```python
from build123d import *

# Parameters (mm, degrees)
F0_R     = 57
F0_R_2   = 55
F1_DEPTH = 65
F3_R     = 2.1
F4_DEPTH = 70
F5_R     = 2.1
F6_DEPTH = 100


with BuildPart() as f1:
    # F0 (on Front) → F1 (new body, symmetric)
    with BuildSketch(Plane.XZ):
        with Locations((11.197514832, 9.3730366789)):
            Circle(F0_R)
        with Locations((11.197514832, 9.3730366789)):
            Circle(F0_R_2, mode=Mode.SUBTRACT)
    extrude(amount=F1_DEPTH, both=True)

    # F3 (on plane+point) → F4 (cut, symmetric)
    with BuildSketch(Plane.YZ.offset(11.197514832)):
        with Locations((0, 9.3730366789)):
            Circle(F3_R)
    extrude(amount=F4_DEPTH, both=True, mode=Mode.SUBTRACT)

    # F5 (on Top) → F6 (cut, symmetric)
    with BuildSketch(Plane.XY):
        with Locations((11.197514832, 0)):
            Circle(F5_R)
    extrude(amount=F6_DEPTH, both=True, mode=Mode.SUBTRACT)


solid = f1.part
```
For this review, take the finished solid that the model builds, in its own axes (mm). Round coordinates to 2 decimals unless told otherwise and drop trailing zeros. Order: outer loops, then holes, each group sorted by start corner. A loop starts at its lowest first (then second) coordinate and runs counter-clockwise, first axis right, second up.
Q1. We need section D-D, the plane y = -22. Give the boundary of the cut face in (x, z).
Findings below:
outline: circle Ø114 at (11.2, 9.37); hole circle Ø110 at (11.2, 9.37)
Q2. Mouldability with a two-part tool opening along X and no side actions: class faces 1 (the cylindrical face through (-1.16, -0.91, -46.27)), 2 (the cylindrical face through (67.192, 1.129, 11.144)), 3 (the cylindrical face through (36.58, 0.91, -39.42)) as pulls with the +X half, pulls with the -X half, needs draft (parallel to the pull), parting line crosses it, or undercut.
Findings below:
face 1: parting line crosses it
face 2: needs draft
face 3: undercut
Q3. We need section B-B, the plane x = 40. Give the boundary of the cut face in (y, z), plus the area to 3 significant figures.
Findings below:
outline: (-65, -39.81) - (65, -39.81) - (65, -37.48) - (-65, -37.48) - close; (-65, 56.23) - (65, 56.23) - (65, 58.56) - (-65, 58.56) - close
area: 606 mm2
Q4. Insertion check: P1, Ø6, axis at y = -9.5, z = 28.5, coming from the +X side; P2, Ø1.5, axis at y = 30, z = 8, coming from the -X side; P3, Ø8, axis at x = -33.5, y = -30.5, coming from the -Z side; P4, Ø3.5, axis at y = 0, z = 9.37, coming from the +X side. Each pin has a flat end and moves straight along its axis. Give the tip position at first contact, or say it passes through.
Findings below:
P1: stops at x = 65.87
P2: stops at x = -45.8
P3: stops at z = -30.54
P4: passes through
Q5. Wall thickness on line 1 (X direction, y = -16.5, z = 8.5); line 2 (X direction, y = -5.5, z = 6.5); line 3 (Z direction, x = 43.5, y = 47.5): over which ranges is each line inside the solid? List them lowest first.
Findings below:
line 1: x = -45.8 to -43.8, 66.19 to 68.19
line 2: x = -45.73 to -43.73, 66.12 to 68.13
line 3: z = -37.59 to -35.14, 53.89 to 56.34
Q6. We need section A-A, the plane z = 28.5. Give the boundary of the cut face in (x, y), plus the area to 3 significant figures.
Findings below:
outline: (-42.5, -65) - (-40.37, -65) - (-40.37, 65) - (-42.5, 65) - close; (62.76, -65) - (64.89, -65) - (64.89, 65) - (62.76, 65) - close
area: 553 mm2
Q7. We need section C-C, the plane y = 0. Give the boundary of the cut face in (x, z).
Findings below:
outline: (-45.76, 7.27) arc R57 ccw to (9.1, -47.59) - (9.1, -45.59) arc R55 cw to (-43.76, 7.27) - close; (-45.76, 11.47) - (-43.76, 11.47) arc R55 cw to (9.1, 64.33) - (9.1, 66.33) arc R57 ccw to start; (13.3, -47.59) arc R57 ccw to (68.16, 7.27) - (66.16, 7.27) arc R55 cw to (13.3, -45.59) - close; (13.3, 64.33) arc R55 cw to (66.16, 11.47) - (68.16, 11.47) arc R57 ccw to (13.3, 66.33) - close
